Design review of the part shown in the three views and the two pictorial views. Dimensions are in mm from the part's minimum x, y and z. A direction names the side the tool comes from. Round coordinates to 2 decimals unless told otherwise and drop trailing zeros. Loops run counter-clockwise (first coordinate to the right, second up) from the corner with the lowest first, then second, coordinate; pieces in that order, holes last. Notation, with made-up numbers: M 26,53.5 L 57,53.5 A21 cw 57,81.5 Z; hole C 53,50.25 d2. An arc over 180 degrees is marked long. One line per question, with ' | ' between items. Start each with the question number.
1) For pin 1 Ø8 at (x, z) = (121, 34.5) entering from +Y, flat-tipped, find the tip position at first contact; note if it passes through.
2) We need section B-B (x = 44.5). Give the boundary of the cut face in (y, z).
3) Mouldability with a two-part tool opening along Z and no side actions: class the marked faces 3, 4, 5 and 6 as pulls with the +Z half, pulls with the -Z half, needs draft (parallel to the pull), parting line crosses it, or undercut.
4) We need section C-C (z = 13.5). Give the boundary of the cut face in (x, y), and give its area (3 significant figures).
5) For probe 1 along X at (y, z) = (47, 33.5); probe 2 along Z at (x, y) = (34, 24); probe 3 along Y at (x, z) = (9, 86), list the stretches that pass through material, from the lowest coordinate up. Write a range as from..to.
6) We need section A-A (y = 67.5). Give the boundary of the cut face in (x, z), and give its area (3 significant figures).
7) For the marked faces 1 and 2, list the 3-axis set-ups (+Z, -Z, +X, -X, +Y, -Y) from which the entire face can be reached by the end or side of a thin tool; tool diameter is ignored.
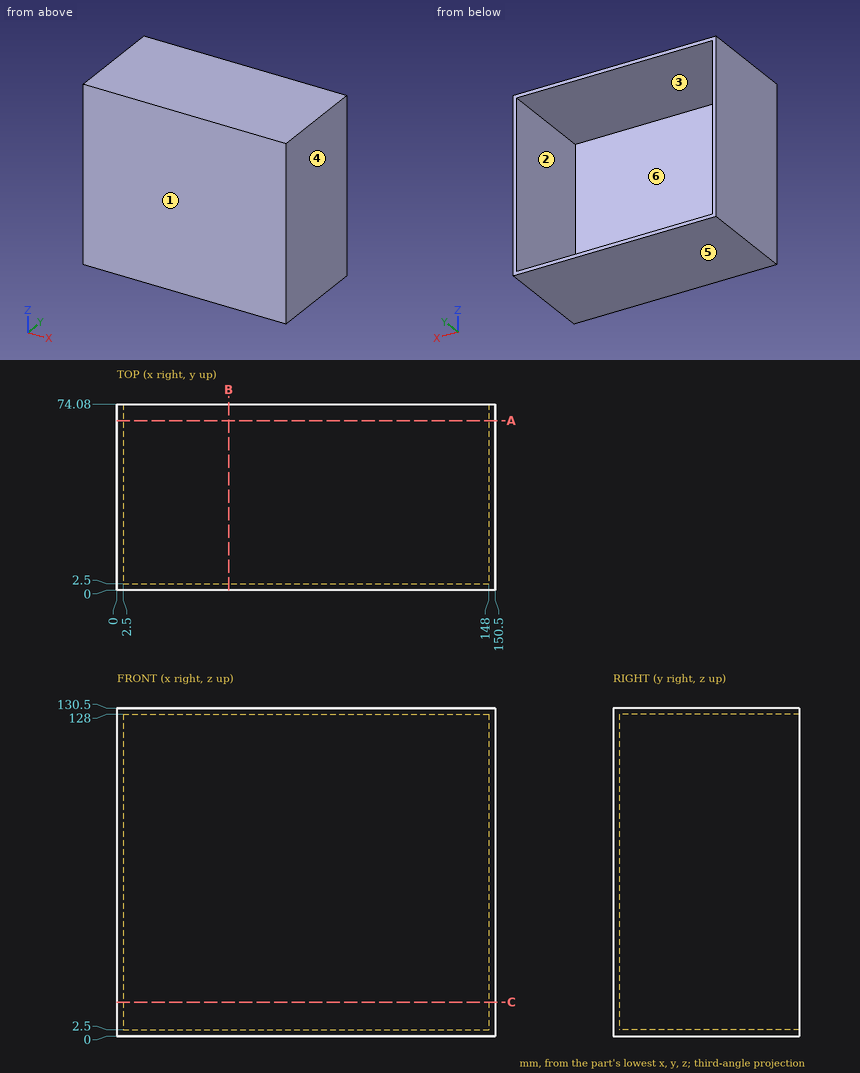
Answers below:
1) pin 1: y = 2.5
2) outline: M 0,0 L 74.08,0 L 74.08,2.5 L 2.5,2.5 L 2.5,128 L 74.08,128 L 74.08,130.5 L 0,130.5 Z
3) face 3: undercut | face 4: needs draft | face 5: pulls with the -Z half | face 6: undercut
4) outline: M 0,0 L 150.5,0 L 150.5,74.08 L 148,74.08 L 148,2.5 L 2.5,2.5 L 2.5,74.08 L 0,74.08 Z | area: 734 mm^2
5) probe 1: 0..2.5, 148..150.5 | probe 2: 0..2.5, 128..130.5 | probe 3: 0..2.5
6) outline: M 0,0 L 150.5,0 L 150.5,130.5 L 0,130.5 Z; hole M 2.5,2.5 L 148,2.5 L 148,128 L 2.5,128 Z | area: 1,380 mm^2
7) face 1: +Z, -Z, +X, -X, -Y | face 2: +Y
